from build123d import *

# Parameters (mm, degrees)
SKETCH1_W                        = 40
SKETCH1_H                        = 20
PCB_DEPTH                        = 1.5
SKETCH3_R                        = 1.5
TOP_MOUNTING_HOLE_DEPTH          = 1.5
SKETCH4_R                        = 1
TOP_MOUNTING_HOLE_2_DEPTH        = 1.5
SKETCH5_R                        = 2.5
SIDE_INLETS_DEPTH                = 1.5
SKETCH6_R                        = 1.5
SIDE_MOUNTING_HOLE_OUTLINE_DEPTH = 1.5
SKETCH7_R                        = 1
SIDE_MOUNTING_HOLES_DEPTH        = 1.5
SKETCH8_R                        = 4.5
SENSOR_BASE_DEPTH                = 0.5
SKETCH9_R                        = 4
SENSOR_DEPTH                     = 7
SENSOR_FILLET_R                  = 0.5
SKETCH10_W                       = 5
SKETCH10_H                       = 12
CONNECTOR_DEPTH                  = 8
SKETCH11_W                       = 4
SKETCH11_H                       = 5
CHIP_DEPTH                       = 1
SKETCH12_R                       = 1.75
BOSS_EXTRUDE10_DEPTH             = 1.2
SKETCH13_W                       = 2
SKETCH13_H                       = 4
BOSS_EXTRUDE11_DEPTH             = 2


with BuildPart() as part:
    # Sketch1 → PCB (new body)
    with BuildSketch(Plane(origin=(0, 0, 0), x_dir=(1, 0, 0), z_dir=(0, 1, 0))):
        Rectangle(SKETCH1_W, SKETCH1_H)
    extrude(amount=PCB_DEPTH)

    # Sketch3 → Top mounting hole (add)
    with BuildSketch(Plane.XZ):
        with Locations((-20, 0)):
            Circle(SKETCH3_R)
    extrude(amount=-TOP_MOUNTING_HOLE_DEPTH)

    # Sketch4 → Top mounting hole 2 (cut)
    with BuildSketch(Plane.XZ):
        with Locations(Location((-20, 0, 0), (0, 0, 270))):
            Circle(SKETCH4_R)
    extrude(amount=-TOP_MOUNTING_HOLE_2_DEPTH, mode=Mode.SUBTRACT)

    # Sketch5 → Side inlets (cut)
    with BuildSketch(Plane.XZ):
        with Locations((-11, -10)):
            Circle(SKETCH5_R)
        with Locations((-11, 10)):
            Circle(SKETCH5_R)
    extrude(amount=-SIDE_INLETS_DEPTH, mode=Mode.SUBTRACT)

    # Sketch6 → side mounting hole outline (add)
    with BuildSketch(Plane(origin=(0, 1.5, 0), x_dir=(1, 0, 0), z_dir=(0, 1, 0))):
        with Locations((10, 10)):
            Circle(SKETCH6_R)
        with Locations((10, -10)):
            Circle(SKETCH6_R)
    extrude(amount=-SIDE_MOUNTING_HOLE_OUTLINE_DEPTH)

    # Sketch7 → side mounting holes (cut)
    with BuildSketch(Plane(origin=(0, 1.5, 0), x_dir=(1, 0, 0), z_dir=(0, 1, 0))):
        with Locations(Location((10, 10, 0), (0, 0, 270))):
            Circle(SKETCH7_R)
        with Locations(Location((10, -10, 0), (0, 0, 270))):
            Circle(SKETCH7_R)
    extrude(amount=-SIDE_MOUNTING_HOLES_DEPTH, mode=Mode.SUBTRACT)

    # Sketch8 → sensor base (add)
    with BuildSketch(Plane(origin=(0, 1.5, 0), x_dir=(1, 0, 0), z_dir=(0, 1, 0))):
        with Locations(Location((-14, 1, 0), (0, 0, 270))):
            Circle(SKETCH8_R)
    extrude(amount=SENSOR_BASE_DEPTH)

    # Sketch9 → sensor (add)
    with BuildSketch(Plane(origin=(0, 2, 0), x_dir=(1, 0, 0), z_dir=(0, 1, 0))):
        with Locations(Location((-14, 1, 0), (0, 0, 270))):
            Circle(SKETCH9_R)
    extrude(amount=SENSOR_DEPTH)

    # sensor fillet
    sensor_fillet_edges = [part.edges().sort_by_distance(p)[0] for p in [
        (-14, 2, -5.5),
        (-14, 9, -5),
    ]]
    fillet(sensor_fillet_edges, radius=SENSOR_FILLET_R - 0.0001)  # a hair under: the kernel refuses the full size

    # Sketch10 → connector (add)
    with BuildSketch(Plane(origin=(0, 1.5, 0), x_dir=(1, 0, 0), z_dir=(0, 1, 0))):
        with Locations((16.5, 0)):
            Rectangle(SKETCH10_W, SKETCH10_H)
    extrude(amount=CONNECTOR_DEPTH)

    # Sketch11 → chip (add)
    with BuildSketch(Plane(origin=(0, 1.5, 0), x_dir=(1, 0, 0), z_dir=(0, 1, 0))):
        with Locations((-2, 5.5)):
            Rectangle(SKETCH11_W, SKETCH11_H)
    extrude(amount=CHIP_DEPTH)

    # Sketch12 → Boss-Extrude10 (add)
    with BuildSketch(Plane(origin=(0, 1.5, 0), x_dir=(1, 0, 0), z_dir=(0, 1, 0))):
        with Locations(Location((0, -1, 0), (0, 0, 270))):
            Circle(SKETCH12_R)
    extrude(amount=BOSS_EXTRUDE10_DEPTH)

    # Sketch13 → Boss-Extrude11 (add)
    with BuildSketch(Plane(origin=(0, 1.5, 0), x_dir=(1, 0, 0), z_dir=(0, 1, 0))):
        with Locations((-2, -5)):
            Rectangle(SKETCH13_W, SKETCH13_H)
    extrude(amount=BOSS_EXTRUDE11_DEPTH)


solid = part.part
Design review of the part built by this model. Coordinates are the model's own, in mm. A direction names the side the tool comes from. Give positions to 0.01 mm unless a question says otherwise; leave off trailing zeros. Order: outer loops, then holes, each group sorted by start corner. A loop starts at its lowest first (then second) coordinate and runs counter-clockwise, first axis right, second up.
1. Add section B-B, the plane y = 7.75. State the section outline as (x, z) points, then the cut area to 3 significant figures.
Solution:
outline: circle Ø8 at (-14, -1); (14, -6) - (19, -6) - (19, 6) - (14, 6) - close
area: 110 mm2
2. For pin 1 Ø2.5 at (y, z) = (6.5, -2.5) entering from +X; pin 2 Ø4 at (x, y) = (-9, 4) entering from -Z; pin 3 Ø5 at (y, z) = (6.5, -9) entering from +X; pin 4 Ø1 at (x, z) = (9.5, 5) entering from +Y, all flat-tipped, find the tip position at first contact; note any pin that passes through.
Solution:
pin 1: stops at x = 19
pin 2: stops at z = -3.65
pin 3: passes through
pin 4: stops at y = 1.5
3. Add section A-A, the plane x = 10. State the section outline as (y, z) points.
Solution:
outline: (0, -11.5) - (1.5, -11.5) - (1.5, -11) - (0, -11) - close; (0, -9) - (1.5, -9) - (1.5, 9) - (0, 9) - close; (0, 11) - (1.5, 11) - (1.5, 11.5) - (0, 11.5) - close
4. Add section C-C, the plane x = 1. State the section outline as (y, z) points.
Solution:
outline: (0, -10) - (1.5, -10) - (1.5, -0.44) - (2.7, -0.44) - (2.7, 2.44) - (1.5, 2.44) - (1.5, 10) - (0, 10) - close
5. Mouldability with a two-part tool opening along Z and no side actions: class faces 1 (the cylindrical face through (-10.9, 0.7, -7.5)), 2 (the flat face through (0, 2.7, 1)), 3 (the cylindrical face through (-21, 1, 0)), 4 (the cylindrical face through (11, 1, -10)) as +Z half, -Z half, draft (parallel to the pull), parting line (faces both ways), or undercut.
Solution:
face 1: -Z half
face 2: draft
face 3: undercut
face 4: undercut
6. To check wall thickness, follow L1, parallel to X at y = 0.8, z = 0; L2, parallel to Z at x = 17, y = 3.75; L3, parallel to X at y = 0.5, z = 10.75. State the ranges of each line that lie inside material, in increasing order.
Solution:
L1: x = -21.5 to -21, -19 to 20
L2: z = -6 to 6
L3: x = 8.7 to 9.34, 10.66 to 11.3
7. Tool access review of faces 5 (the flat face through (-2, 2, 7)), 6 (the flat face through (-2, 3.5, 5)), 7 (the flat face through (-17, 1, -10)): name each direction out of +Z, -Z, +X, -X, +Y, -Y from which nothing blocks a thin tool from reaching the whole face with its end or side.
Solution:
face 5: +Z, +X, -X, +Y
face 6: +Z, -Z, -X, +Y
face 7: -Z, -X, +Y, -Y
